For this review, take the finished solid that the model builds, in its own axes (mm). Give positions to 0.01 mm unless a question says otherwise; leave off trailing zeros. Loops run counter-clockwise (first coordinate to the right, second up) from the corner with the lowest first, then second, coordinate; pieces in that order, holes last.
```python
from build123d import *

# Parameters (mm, degrees)
CROQUIS1_W                                 = 120
CROQUIS1_H                                 = 16
SALIENTE_EXTRUIR1_DEPTH                    = 10
PERFORADOR_PARA_ROSCAR_PARA_MACHO_DE_ROS_D = 4.2
TALADRO_DE_MARGEN_PARA_1_41_D              = 6.7564


with BuildPart() as part:
    # Croquis1 → Saliente-Extruir1 (new body)
    with BuildSketch(Plane.XY):
        with Locations((20.530427632, 3.875)):
            Rectangle(CROQUIS1_W, CROQUIS1_H)
    extrude(amount=SALIENTE_EXTRUIR1_DEPTH)

    # Perforador para roscar para macho de roscar para M5x0.81 (through all)
    with Locations(Plane.XY.offset(10)):
        with Locations((-9.469572368, 3.875), (50.530427632, 3.875)):
            Hole(PERFORADOR_PARA_ROSCAR_PARA_MACHO_DE_ROS_D / 2)

    # Taladro de margen para 1/41 (through all)
    with Locations(Plane.XY.offset(10)):
        with Locations((-24.469572368, 3.554018425), (20.530427632, 3.691581957), (65.530427632, 3.829145489)):
            Hole(TALADRO_DE_MARGEN_PARA_1_41_D / 2)


solid = part.part
```
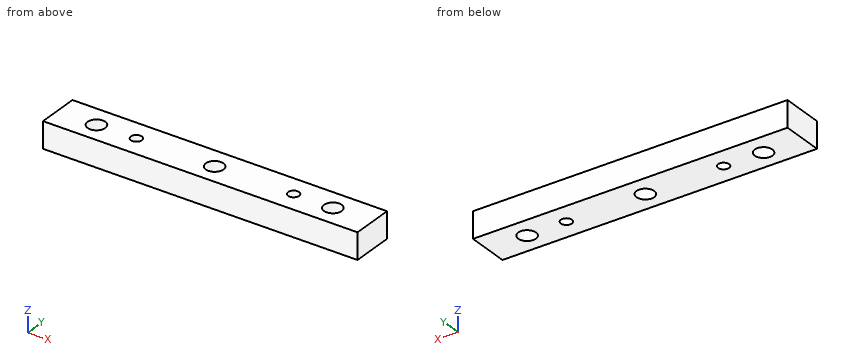
Q1. For probe 1 along Y at (x, z) = (19.5, 5) (3 decimals); probe 2 along X at (y, z) = (4.5, 0.75); probe 3 along Y at (x, z) = (20.5, 7.5) (3 decimals), list the stretches that pass through material, from the lowest coordinate up.
Answers:
probe 1: y = -4.125 to 0.474, 6.909 to 11.875
probe 2: x = -39.47 to -27.71, -21.23 to -11.47, -7.46 to 17.25, 23.81 to 48.53, 52.54 to 62.22, 68.84 to 80.53
probe 3: y = -4.125 to 0.314, 7.07 to 11.875
Q2. Consider section C-C on x = 51.5. Give the boundary of the cut face in (y, z) (3 decimals).
Answers:
outline: (-4.125, 0) - (2.012, 0) - (2.012, 10) - (-4.125, 10) - close; (5.738, 0) - (11.875, 0) - (11.875, 10) - (5.738, 10) - close
Q3. Consider section B-B on x = 67. Give the boundary of the cut face in (y, z) (3 decimals), plus the area to 3 significant figures.
Answers:
outline: (-4.125, 0) - (0.787, 0) - (0.787, 10) - (-4.125, 10) - close; (6.871, 0) - (11.875, 0) - (11.875, 10) - (6.871, 10) - close
area: 99.2 mm2
Q4. For pin 1 Ø2.5 at (x, y) = (-9.47, 3.88) entering from +Z, flat-tipped, find the tip position at first contact; note if it passes through.
Answers:
pin 1: passes through
Q5. Consider section A-A on z = 1.75. Give the boundary of the cut face in (x, y) (3 decimals).
Answers:
outline: (-39.47, -4.125) - (80.53, -4.125) - (80.53, 11.875) - (-39.47, 11.875) - close; hole circle Ø6.756 at (-24.47, 3.554); hole circle Ø4.2 at (-9.47, 3.875); hole circle Ø6.756 at (20.53, 3.692); hole circle Ø4.2 at (50.53, 3.875); hole circle Ø6.756 at (65.53, 3.829)
